Can you work these out from the model? Positions are in its coordinate system, mm. A direction names the side the tool comes from. Give positions to 0.01 mm unless a question says otherwise; leave off trailing zeros. Order: outer loops, then holes, each group sorted by start corner. A loop starts at its lowest first (then second) coordinate and runs counter-clockwise, first axis right, second up.
Item 1: I want a section at B-B, the plane y = -52. Write out the boundary of the cut face in (x, z), then the cut area to 3 significant figures.
Item 2: I want a section at A-A, the plane z = 6.75. Write out the boundary of the cut face in (x, y), then the cut area to 3 significant figures.
Item 3: If I drill on line 1 along Y through (x, z) = (-13, 1.25); line 2 along Y through (x, z) = (-7, 10); line 3 along X through (y, z) = (-60, 7), over which ranges is the centre line in solid material (lowest first)?
Item 4: If we mould it in two halves opening along X, with no side actions, what happens to faces 6 (the flat face through (1.137, -57, -1)), 7 (the flat face through (-26.863, -57, -1)), 8 (the flat face through (-13, -25, 0)), 9 (the flat face through (-13, -59.212, 2))? For each: +X half, -X half, draft (parallel to the pull), parting line (faces both ways), or undercut.
Item 5: I'm going to push flat-ended pins straight in: pin 1 Ø6 at (x, y) = (-14, -54) entering from -Z; pin 2 Ø2 at (x, y) = (-8.5, -24) entering from +Z; pin 3 Ø8.5 at (x, y) = (-11.5, -42) entering from -Z; pin 4 Ø5 at (y, z) = (-47, 4.5) entering from +X. Where does each tip first touch, or does it pass through?
Item 6: I want a section at C-C, the plane z = -0.75. Write out the boundary of the cut face in (x, y).
Item 7: I want a section at D-D, the plane x = -18.5. Write out the boundary of the cut face in (y, z).
Item 8: Which directions (+Z, -Z, +X, -X, +Y, -Y) give clear straight access to the entire face, cutting with the end or side of a thin tool? Please do faces 1 (the flat face through (-13, -58, -4)), 2 (the flat face through (-13, -63, 1)), 3 (the flat face through (-26, -56, 3)), 4 (the flat face through (-13, -44, 0)), 5 (the flat face through (-13, -67.712, 5)).
```python
from build123d import *

# Parameters (mm, degrees)
SKETCH_1_W          = 24
SKETCH_1_H          = 47
EXTRUDE_1_DEPTH     = 11
SKETCH_2_W          = 21
SKETCH_2_H          = 44
CUT_EXTRUDE_1_DEPTH = 10
SKETCH_3_W          = 6.5
SKETCH_3_H          = 6.352849337
EXTRUDE_2_DEPTH     = 26
SKETCH_4_W          = 7
SKETCH_4_H          = 6.352849337
EXTRUDE_3_DEPTH     = 2
CUT_EXTRUDE_2_DEPTH = 35


with BuildPart() as part:
    # 草图1 → 凸台-拉伸1 (new body)
    with BuildSketch(Plane.XY):
        with Locations((-12.862884841, -44.211686375)):
            Rectangle(SKETCH_1_W, SKETCH_1_H)
    extrude(amount=EXTRUDE_1_DEPTH)

    # 草图2 → 切除-拉伸1 (cut)
    with BuildSketch(Plane.XY.offset(11)):
        with Locations((-12.862884841, -44.211686375)):
            Rectangle(SKETCH_2_W, SKETCH_2_H)
    extrude(amount=-CUT_EXTRUDE_1_DEPTH, mode=Mode.SUBTRACT)

    # 草图3 → 凸台-拉伸2 (add)
    with BuildSketch(Plane.ZY.offset(24.862884841)):
        with Locations((-0.75, -32.388111044)):
            Rectangle(SKETCH_3_W, SKETCH_3_H)
        with Locations((-0.75, -56.035261707)):
            Rectangle(SKETCH_3_W, SKETCH_3_H)
    extrude(amount=-EXTRUDE_2_DEPTH)

    # 草图4 → 凸台-拉伸3 (add)
    with BuildSketch(Plane.ZY.offset(24.862884841)):
        with Locations((-0.5, -32.388111044)):
            Rectangle(SKETCH_4_W, SKETCH_4_H)
        with Locations((-0.5, -56.035261707)):
            Rectangle(SKETCH_4_W, SKETCH_4_H)
    extrude(amount=EXTRUDE_3_DEPTH)

    # 草图6 → 切除-拉伸2 (cut)
    with BuildSketch(Plane.ZY.offset(26.862884841)):
        Polygon((0, -35.564535712), (-4, -32.388111043), (-4, -35.564535712), align=None)
        Polygon((0, -52.858837038), (-4, -56.035261706), (-4, -52.858837038), align=None)
    extrude(amount=-CUT_EXTRUDE_2_DEPTH, mode=Mode.SUBTRACT)


solid = part.part
```
Results list:
1. outline: (-24.86, 0) - (-0.86, 0) - (-0.86, 11) - (-2.36, 11) - (-2.36, 1) - (-23.36, 1) - (-23.36, 11) - (-24.86, 11) - close
1. area: 54.0 mm2
2. outline: (-24.86, -67.71) - (-0.86, -67.71) - (-0.86, -20.71) - (-24.86, -20.71) - close; hole (-23.36, -66.21) - (-2.36, -66.21) - (-2.36, -22.21) - (-23.36, -22.21) - close
2. area: 204 mm2
3. line 1: y = -67.71 to -66.21, -59.21 to -52.86, -35.56 to -29.21, -22.21 to -20.71
3. line 2: y = -67.71 to -66.21, -22.21 to -20.71
3. line 3: x = -24.86 to -23.36, -2.36 to -0.86
4. face 6: +X half
4. face 7: -X half
4. face 8: draft
4. face 9: undercut
5. pin 1: stops at z = -4
5. pin 2: stops at z = 1
5. pin 3: stops at z = 0
5. pin 4: stops at x = -0.86
6. outline: (-26.86, -59.21) - (1.14, -59.21) - (1.14, -53.45) - (-26.86, -53.45) - close; (-26.86, -34.97) - (1.14, -34.97) - (1.14, -29.21) - (-26.86, -29.21) - close
7. outline: (-67.71, 0) - (-59.21, 0) - (-59.21, -4) - (-56.04, -4) - (-52.86, 0) - (-35.56, 0) - (-32.39, -4) - (-29.21, -4) - (-29.21, 0) - (-20.71, 0) - (-20.71, 11) - (-22.21, 11) - (-22.21, 1) - (-29.21, 1) - (-29.21, 2.5) - (-35.56, 2.5) - (-35.56, 1) - (-52.86, 1) - (-52.86, 2.5) - (-59.21, 2.5) - (-59.21, 1) - (-66.21, 1) - (-66.21, 11) - (-67.71, 11) - close
8. face 1: -Z, +X, -X, +Y, -Y
8. face 2: +Z
8. face 3: +Z, -X, +Y, -Y
8. face 4: -Z, +X, -X
8. face 5: +Z, -Z, +X, -X, -Y
